from build123d import *

# Parameters (mm, degrees)
EXTRUDE_1_DEPTH     = 5
FILLET_2_R          = 1
HOLE_WIZARD_M3_1_D  = 2.5
SKETCH_5_R          = 5
CUT_EXTRUDE_1_DEPTH = 5
HOLE_WIZARD_M5_1_D  = 4.2
SKETCH_7_R          = 10
CUT_EXTRUDE_2_DEPTH = 78.99358948
SKETCH_8_R          = 19
CUT_EXTRUDE_3_DEPTH = 1


with BuildPart() as part:
    # 草图1 → 凸台-拉伸1 (new body)
    with BuildSketch(Plane.XY):
        Polygon((-57, 35), (-57, -35), (-12, -35), (-12, -53), (12, -53), (12, -35), (57, -35), (57, 35), (12, 35), (12, 53), (-12, 53), (-12, 35), align=None)
    extrude(amount=EXTRUDE_1_DEPTH)

    # 圆角2
    fillet_2_edges = [part.edges().sort_by_distance(p)[0] for p in [
        (-12, 53, 2.5),
        (12, 53, 2.5),
        (57, 35, 2.5),
        (57, -35, 2.5),
        (12, -53, 2.5),
        (-12, -53, 2.5),
        (-57, -35, 2.5),
        (-57, 35, 2.5),
    ]]
    fillet(fillet_2_edges, radius=FILLET_2_R)

    # M3 螺纹孔的螺纹孔钻头1 (through all)
    with Locations(Plane(origin=(-23.5, 30.5, 5), x_dir=(1, 0, 0), z_dir=(0, 0, 1))):
        with Locations((0, 0), (0, -47)):
            hole_wizard_m3_1 = Hole(HOLE_WIZARD_M3_1_D / 2)

    # 镜向1: M3 螺纹孔的螺纹孔钻头1 across plane
    add(hole_wizard_m3_1.mirror(Plane(origin=(0, 0, 0), x_dir=(0, 0, 1), z_dir=(1, 0, 0))), mode=Mode.SUBTRACT)

    # 草图5 → 切除-拉伸1 (cut)
    with BuildSketch(Plane.XY.offset(5)):
        with Locations((-48, 26)):
            Circle(SKETCH_5_R)
        with Locations((-48, -26)):
            Circle(SKETCH_5_R)
    cut_extrude_1 = extrude(amount=-CUT_EXTRUDE_1_DEPTH, mode=Mode.SUBTRACT)

    # 镜向2: 切除-拉伸1 across plane
    add(cut_extrude_1.mirror(Plane(origin=(0, 0, 0), x_dir=(0, 0, 1), z_dir=(1, 0, 0))), mode=Mode.SUBTRACT)

    # M5 螺纹孔的螺纹孔钻头1 (through all)
    with Locations(Plane(origin=(0, 45.5, 5), x_dir=(1, 0, 0), z_dir=(0, 0, 1))):
        with Locations((0, 0)):
            hole_wizard_m5_1 = Hole(HOLE_WIZARD_M5_1_D / 2)

    # 镜向3: M5 螺纹孔的螺纹孔钻头1 across plane
    add(hole_wizard_m5_1.mirror(Plane.ZX), mode=Mode.SUBTRACT)

    # 草图7 → 切除-拉伸2 (cut, through all)
    with BuildSketch(Plane.XY.offset(5)):
        with Locations((0, 7)):
            Circle(SKETCH_7_R)
    extrude(amount=-CUT_EXTRUDE_2_DEPTH, mode=Mode.SUBTRACT)

    # 草图8 → 切除-拉伸3 (cut)
    with BuildSketch(Plane.XY.offset(5)):
        with Locations((0, 7)):
            Circle(SKETCH_8_R)
    extrude(amount=-CUT_EXTRUDE_3_DEPTH, mode=Mode.SUBTRACT)


solid = part.part
Build history of the part. All positions in model axes, mm. A direction names the side the tool comes from. Round coordinates to 2 decimals unless told otherwise and drop trailing zeros. Loops run counter-clockwise (first coordinate to the right, second up) from the corner with the lowest first, then second, coordinate; pieces in that order, holes last. Notation, with made-up numbers: (86.5, 56) -> (112.5, 56) arc R17 ccw to (112.5, 82) -> close; hole circle Ø11 at (-12.5, 22). An arc over 180 degrees is marked (long way). Use CSV: the item, a comma, the result in double quotes. Start each with the question number.
Q1. Saw through at D-D on x = 0. Give the cut face in (y, z), and give its area (3 significant figures).
Q2. Flat gauge pins, fed straight in: pin 1 Ø12 at (x, y) = (37.5, 30) entering from -Z; pin 2 Ø1.5 at (y, z) = (-37, 3) entering from +X; pin 3 Ø1.5 at (y, z) = (47.5, 2) entering from -X; pin 4 Ø2.5 at (x, z) = (-27.5, 3) entering from -Y. Where does each tip first touch, or does it go through?
Q3. Saw through at C-C on y = -26. Give the cut face in (x, z).
Q4. Drill centre lines: L1, parallel to Y at x = -48.5, z = 1.85; L2, parallel to Y at x = 0, z = 4.7; L3, parallel to Y at x = 0, z = 3.65. Where is each one in solid material? Low to high.
Q5. Which spindle directions (+Z, -Z, +X, -X, +Y, -Y) get a long thin tool onto all of the face, cutting with end or side? Do faces 1 (the face through (12, 43, 2)), 2 (the face through (0, 53, 2)), 3 (the face through (8, -1, 4)), 4 (the face through (34, -35, 2)), 5 (the face through (24.172, -15.446, 2.465)). Say none if no direction does.
Q6. Saw through at A-A on y = 7. Give the cut face in (x, z), and give its area (3 significant figures).
Q7. Saw through at B-B on x = -23.5. Give the cut face in (y, z), and give its area (3 significant figures).
Q8. Mould opens along Y. For faces 6 (the face through (-34, 35, 2)), 7 (the face through (-52, 23, 3)), 8 (the face through (0, -53, 2)) say: +Y half, -Y half, draft (parallel to the pull), parting line (faces both ways), or undercut.
Solutions:
1,outline,"(-53, 0) -> (-47.6, 0) -> (-47.6, 5) -> (-53, 5) -> close; (-43.4, 0) -> (-3, 0) -> (-3, 4) -> (-12, 4) -> (-12, 5) -> (-43.4, 5) -> close; (17, 0) -> (43.4, 0) -> (43.4, 5) -> (26, 5) -> (26, 4) -> (17, 4) -> close; (47.6, 0) -> (53, 0) -> (53, 5) -> (47.6, 5) -> close"
1,area,"370 mm^2"
2,pin 1,"stops at z = 0"
2,pin 2,"stops at x = 12"
2,pin 3,"stops at x = -12"
2,pin 4,"stops at y = -35"
3,outline,"(-57, 0) -> (-53, 0) -> (-53, 5) -> (-57, 5) -> close; (-43, 0) -> (43, 0) -> (43, 5) -> (-43, 5) -> close; (53, 0) -> (57, 0) -> (57, 5) -> (53, 5) -> close"
4,L1,"y = -35 to -30.97, -21.03 to 21.03, 30.97 to 35"
4,L2,"y = -53 to -47.6, -43.4 to -12, 26 to 43.4, 47.6 to 53"
4,L3,"y = -53 to -47.6, -43.4 to -3, 17 to 43.4, 47.6 to 53"
5,face 1,"+Z, -Z, +X, +Y"
5,face 2,"+Z, -Z, +X, -X, +Y"
5,face 3,"+Z"
5,face 4,"+Z, -Z, +X, -Y"
5,face 5,"+Z, -Z"
6,outline,"(-57, 0) -> (-10, 0) -> (-10, 4) -> (-19, 4) -> (-19, 5) -> (-57, 5) -> close; (10, 0) -> (57, 0) -> (57, 5) -> (19, 5) -> (19, 4) -> (10, 4) -> close"
6,area,"452 mm^2"
7,outline,"(-35, 0) -> (-17.75, 0) -> (-17.75, 5) -> (-35, 5) -> close; (-15.25, 0) -> (29.25, 0) -> (29.25, 5) -> (-15.25, 5) -> close; (31.75, 0) -> (35, 0) -> (35, 5) -> (31.75, 5) -> close"
7,area,"325 mm^2"
8,face 6,"+Y half"
8,face 7,"undercut"
8,face 8,"-Y half"
